Design review of the part shown in the three views and the two pictorial views. Dimensions are in mm from the part's minimum x, y and z. A direction names the side the tool comes from. Round coordinates to 2 decimals unless told otherwise and drop trailing zeros. Write each loop counter-clockwise with the first axis right and the second up, starting at its lowest first coordinate (ties: lowest second). Pieces come first, ordered by that corner, then holes. Notation, with made-up numbers: (44.25, 11) -> (65.25, 11) arc R6 ccw to (65.25, 18) -> close; hole circle Ø8 at (73.5, 23). An arc over 180 degrees is marked (long way). Return JSON: item names as keys, results as strings. Group by question number.
1. Take a section at C-C, the plane z = 9. Write out the cut boundary in (x, y).
2. Clearance check with flat-ended pins moving along their axes: P1, Ø3, axis at y = 14.5, z = 8, coming from the -X side; P2, Ø6.5, axis at x = 10, z = 3.5, coming from the +Y side; P3, Ø2, axis at x = 24.5, y = 5.5, coming from the +Z side. State where each tip first meets the part, or that it passes through.
3. For line 1 along Z through (x, y) = (11, 6.5); line 2 along Y through (x, z) = (12.5, 12); line 3 along X through (y, z) = (5, 11.25), list the stretches that pass through material, from the lowest coordinate up. Write a range as from..to.
4. Tool access review of the marked faces 5, 6 and 7: name each direction out of +Z, -Z, +X, -X, +Y, -Y from which nothing blocks a thin tool from reaching the whole face with its end or side.
5. Mouldability with a two-part tool opening along X and no side actions: class the marked faces 1, 2, 3 and 4 as pulls with the +X half, pulls with the -X half, needs draft (parallel to the pull), parting line crosses it, or undercut.
6. Take a section at D-D, the plane x = 28. Write out the cut boundary in (y, z), then the cut area to 3 significant figures.
7. Take a section at A-A, the plane z = 1.5. Write out the cut boundary in (x, y).
8. Take a section at B-B, the plane x = 11. Write out the cut boundary in (y, z).
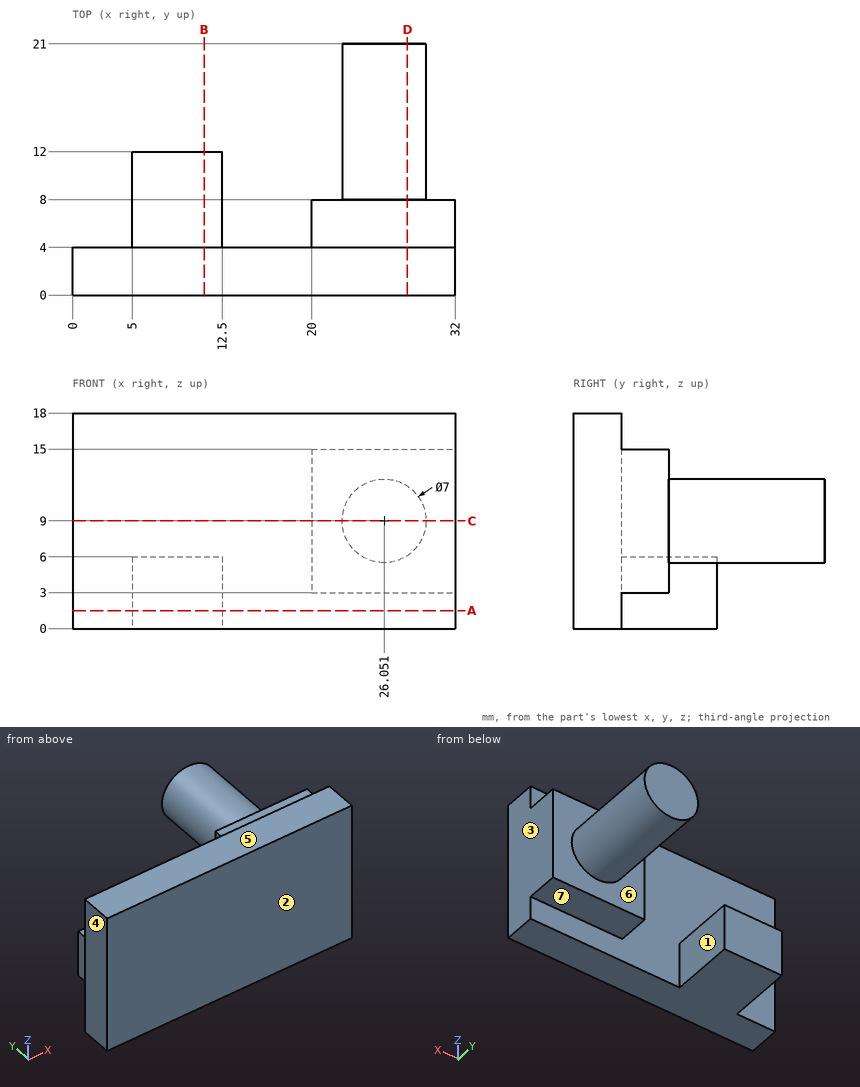
Output:
{
 "1": {"outline": "(0, 0) -> (32, 0) -> (32, 8) -> (29.55, 8) -> (29.55, 21) -> (22.55, 21) -> (22.55, 8) -> (20, 8) -> (20, 4) -> (0, 4) -> close"},
 "2": {"P1": "stops at x = 22.55", "P2": "stops at y = 12", "P3": "stops at z = 15"},
 "3": {"line 1": "z = 0..6", "line 2": "y = 0..4", "line 3": "x = 20..32"},
 "4": {"face 5": "+Z, +X, -X, +Y, -Y", "face 6": "+Y", "face 7": "-Z, +X, +Y"},
 "5": {"face 1": "undercut", "face 2": "needs draft", "face 3": "pulls with the +X half", "face 4": "pulls with the -X half"},
 "6": {"outline": "(0, 0) -> (4, 0) -> (4, 3) -> (8, 3) -> (8, 6.09) -> (21, 6.09) -> (21, 11.91) -> (8, 11.91) -> (8, 15) -> (4, 15) -> (4, 18) -> (0, 18) -> close", "area": "196 mm^2"},
 "7": {"outline": "(0, 0) -> (32, 0) -> (32, 4) -> (12.5, 4) -> (12.5, 12) -> (5, 12) -> (5, 4) -> (0, 4) -> close"},
 "8": {"outline": "(0, 0) -> (12, 0) -> (12, 6) -> (4, 6) -> (4, 18) -> (0, 18) -> close"}
}
